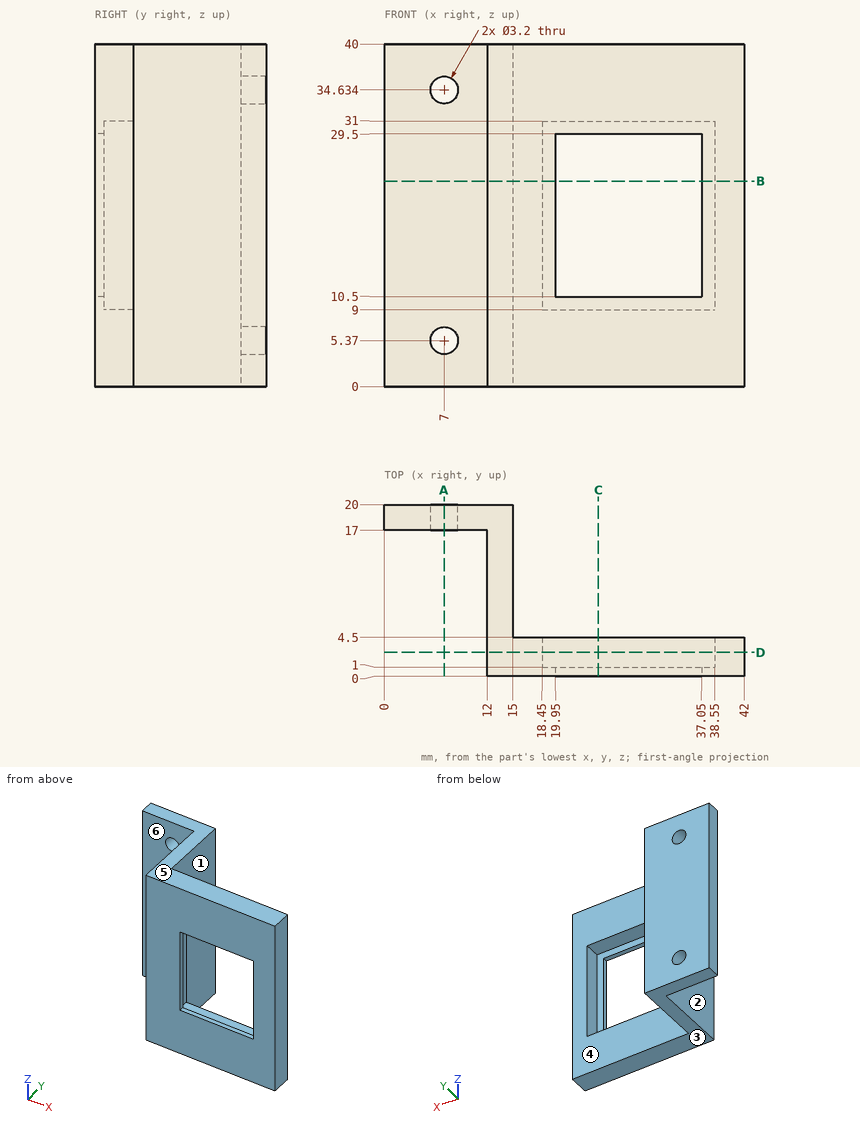
Here's the drawing with two shaded views (mm, measured from the low corner). I have some questions. A direction names the side the tool comes from. Give positions to 0.01 mm unless a question says otherwise; leave off trailing zeros. Order: outer loops, then holes, each group sorted by start corner. A loop starts at its lowest first (then second) coordinate and runs counter-clockwise, first axis right, second up. Notation, with made-up numbers: (10, 73.25) -> (44, 73.25) arc R22 cw to (44, 102.25) -> close; hole circle Ø4 at (1.25, 46.5). An arc over 180 degrees is marked (long way). Use a Markdown table: item, result. Add a question column.
Item 1: For the marked faces 4, 5 and 6, which set-ups out of +Z, -Z, +X, -X, +Y, -Y let a thin tool reach every point of the face, with its end or its side?
Item 2: Imagine slicing it at C-C on x = 25. Please give me the cut outline in (y, z), plus the area to 3 significant figures.
Item 3: Imagine slicing it at A-A on x = 7. Please give me the cut outline in (y, z), plus the area to 3 significant figures.
Item 4: I need wall thicknesses on line 1 (Z direction, x = 23, y = 1.5); line 2 (Y direction, x = 4.5, z = 18); line 3 (Y direction, x = 16, z = 30). Which ranges of each line are inside material? Lowest first, please.
Item 5: Imagine slicing it at B-B on z = 24. Please give me the cut outline in (x, y).
Item 6: If we mould it in two halves opening along X, with no side actions, what happens to the marked faces 1, 2 and 3? For each: pulls with the +X half, pulls with the -X half, needs draft (parallel to the pull), parting line crosses it, or undercut.
Item 7: Will these pins go through, and if not, where does the flat tip stop? pin 1 (1 mm diameter, centred on x = 36.5, z = 7, fed in from +Y); pin 2 (1.9 mm diameter, centred on x = 7, z = 34.634, fed in from +Y); pin 3 (2 mm diameter, centred on y = 15.5, z = 11, fed in from +X); pin 4 (6 mm diameter, centred on y = 11.5, z = 22.5, fed in from -X).
Item 8: Imagine slicing it at D-D on y = 2.75. Please give me the cut outline in (x, z).
Data:
| question | item | result |
|---|---|---|
| 1 | face 4 | +Z, -Z, +X, +Y |
| 1 | face 5 | +Z, +X, -X, +Y, -Y |
| 1 | face 6 | +Z, -Z, -X, -Y |
| 2 | outline | (0, 0) -> (4.5, 0) -> (4.5, 9) -> (1, 9) -> (1, 10.5) -> (0, 10.5) -> close; (0, 29.5) -> (1, 29.5) -> (1, 31) -> (4.5, 31) -> (4.5, 40) -> (0, 40) -> close |
| 2 | area | 84.0 mm² |
| 3 | outline | (17, 0) -> (20, 0) -> (20, 3.77) -> (17, 3.77) -> close; (17, 6.97) -> (20, 6.97) -> (20, 33.03) -> (17, 33.03) -> close; (17, 36.23) -> (20, 36.23) -> (20, 40) -> (17, 40) -> close |
| 3 | area | 101 mm² |
| 4 | line 1 | z = 0 to 9, 31 to 40 |
| 4 | line 2 | y = 17 to 20 |
| 4 | line 3 | y = 0 to 4.5 |
| 5 | outline | (0, 17) -> (12, 17) -> (12, 0) -> (19.95, 0) -> (19.95, 1) -> (18.45, 1) -> (18.45, 4.5) -> (15, 4.5) -> (15, 20) -> (0, 20) -> close; (37.05, 0) -> (42, 0) -> (42, 4.5) -> (38.55, 4.5) -> (38.55, 1) -> (37.05, 1) -> close |
| 6 | face 1 | pulls with the +X half |
| 6 | face 2 | pulls with the -X half |
| 6 | face 3 | needs draft |
| 7 | pin 1 | stops at y = 4.5 |
| 7 | pin 2 | passes through |
| 7 | pin 3 | stops at x = 15 |
| 7 | pin 4 | stops at x = 12 |
| 8 | outline | (12, 0) -> (42, 0) -> (42, 40) -> (12, 40) -> close; hole (18.45, 9) -> (38.55, 9) -> (38.55, 31) -> (18.45, 31) -> close |
